```python
from build123d import *

# Parameters (mm, degrees)
F0_R      = 12.7
F1_DEPTH  = 76.2
F1_FACE_R = 12.7
F2_DEPTH  = 25.4
F2_TAPER  = 30
F3_T      = -2.54
F5_DEPTH  = 1.27
F6_SIZE   = 1.2699
F7_COUNT  = 8


# Not quite as in the source:
# - a fillet or chamfer is up to 0.001 mm smaller than in the source, because OpenCascade refuses the exact size


with BuildPart() as f1:
    # F0 (on Top) → F1 (new body)
    with BuildSketch(Plane.XY):
        Circle(F0_R)
    extrude(amount=F1_DEPTH)

    # F1_face (on face) → F2 (join)
    with BuildSketch(Plane.XY.offset(76.2)):
        Circle(F1_FACE_R)
    extrude(amount=F2_DEPTH, taper=F2_TAPER)

    # F3
    f3_openings = [f1.faces().sort_by_distance(p)[0] for p in [
        (0, 0, 0),
    ]]
    offset(amount=F3_T, openings=f3_openings)

    # F4 (on Front) → F5 (join, symmetric)
    with BuildSketch(Plane.XZ):
        Polygon((-11.43, 25.4), (-36.83, 0), (-11.43, 0), align=None)
    extrude(amount=F5_DEPTH, both=True)

    # F6 (size 1.27 in the source; OpenCascade refuses exactly that, so slightly less here)
    f6_edges = [f1.edges().sort_by_distance(p)[0] for p in [
        (-24.73317, -1.27, 12.09683),
        (-24.73317, 1.27, 12.09683),
    ]]
    chamfer(f6_edges, length=F6_SIZE)

    # F7: F1 ×8 about axis
    f7_axis = Axis((0, 0, 0), (0, 0, 1))


with BuildPart() as f1_1:
    add(f1.part)
    for i in range(1, F7_COUNT):
        add(f1.part.rotate(f7_axis, i * 360 / F7_COUNT))


solid = f1_1.part
```
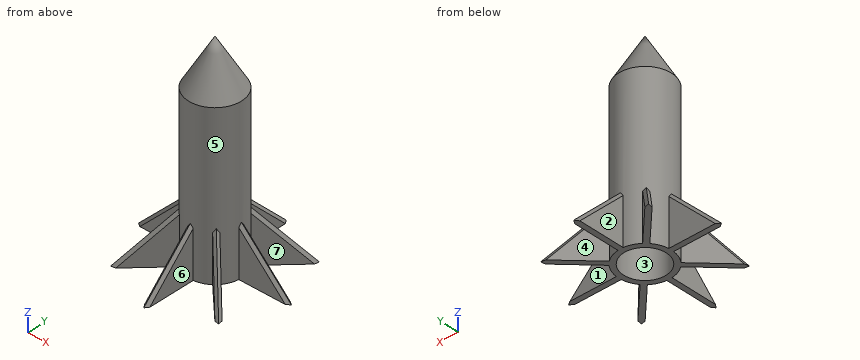
Work out the finished part from the listing and answer in its coordinate system (mm). Face numbers are marked on the shaded views. A direction names the side the tool comes from. Give positions to 0.01 mm unless a question says otherwise; leave off trailing zeros. Loops run counter-clockwise (first coordinate to the right, second up) from the corner with the lowest first, then second, coordinate; pieces in that order, holes last. Notation, with made-up numbers: (31, 16.5) -> (75, 16.5) arc R33 cw to (75, 48.5) -> close; hole circle Ø11 at (-9.75, -12). An arc over 180 degrees is marked (long way). One line per question, with ' | ' between items. Start each with the question number.
1) Determine the mould class of the marked faces 1, 2, 3 and 4 for opening direction Y: +Y half, -Y half, draft (parallel to the pull), parting line (faces both ways), or undercut.
2) Section A-A, the plane y = -18.5 is taken. State how many separate pieces and enclosed holes the cut face has, then the cut area to 3 significant figures.
3) For the marked faces 5, 6 and 7, determine the directions among +Z, -Z, +X, -X, +Y, -Y from which every point of the face is accessible in a straight line to the end or side of a thin tool.
4) Section B-B, the plane z = 49.5 is taken. Determine the outline of the cut face in (x, y), then the cut area to 3 significant figures.
5) Each of these flat-tipped pins is pushed along its axis until it touches: pin 1 (1.5 mm diameter, centred on x = -13, z = 17, fed in from +Y); pin 2 (6 mm diameter, centred on y = -11.5, z = 19.5, fed in from +X); pin 3 (18 mm diameter, centred on y = -26, z = 14, fed in from -X); pin 4 (3 mm diameter, centred on x = 15.5, z = 59, fed in from +Y). Where does it stop, or does it pass through?
6) Straight lines are drawn through the part: L1, parallel to Y at x = 0, z = 29; L2, parallel to X at y = 0.5, z = 28.5; L3, parallel to Z at x = 8, y = 0. For each, find the intervals that lie inside material, in ascending order.
Resolved:
1) face 1: undercut | face 2: draft | face 3: undercut | face 4: +Y half
2) separate pieces: 3 | enclosed holes: 0 | area: 114 mm2
3) face 5: +Z | face 6: +Z, -Z, -Y | face 7: +Z, -Z, +X
4) outline: circle Ø25.4 at (0, 0); hole circle Ø20.32 at (0, 0) | area: 182 mm2
5) pin 1: y = 14.3 | pin 2: x = 13.96 | pin 3: x = -21.75 | pin 4: through
6) L1: -12.7 to -10.16, 10.16 to 12.7 | L2: -12.69 to -10.15, 10.15 to 12.69 | L3: 79.26 to 84.34
